Verification items for the finished model (mm, model axes). Coordinates: 2 decimals unless noted, no trailing zeros. Order: outer loops, then holes, each group sorted by start corner. A loop starts at its lowest first (then second) coordinate and runs counter-clockwise, first axis right, second up.
Q1. Cross-section at D-D, the plane x = -8.5. Record the boundary of the cut face in (y, z), and give its area (3 significant figures).
Q2. Cross-section at C-C, the plane y = 0.75. Record the boundary of the cut face in (x, z).
Q3. Thickness scan on line 1 (Y direction, x = 6, z = 6.5); line 2 (X direction, y = 1, z = 1.25); line 3 (X direction, y = 4.25, z = 1.5). Record the ranges inside material, lowest first.
Q4. Cross-section at B-B, the plane z = 8.5. Record the boundary of the cut face in (x, y), and give its area (3 significant figures).
Q5. Cross-section at A-A, the plane z = 5.75. Record the boundary of the cut face in (x, y).
Q6. Draft check along X on faces 1 (the conical face through (-4.59, -10.975, 9.604)), 2 (the flat face through (0, 0, 8)), 3 (the flat face through (5, -5, 0)), 4 (the conical face through (4.59, 10.975, 0.396)). Enter one of: pulls with the +X half, pulls with the -X half, needs draft (parallel to the pull), parting line crosses it, or undercut.
Q7. Depth check by flat-ended pin: P1, Ø4, axis at x = 0, y = -3, coming from the -Z side; P2, Ø1, axis at y = -7.5, z = 7, coming from the -X side; P3, Ø1.5, axis at y = 9, z = 3, coming from the -X side. Enter the tip coordinate at first touch or a pass-through.
from build123d import *

# Parameters (mm, degrees)
F1_DEPTH = 10
F2_DEPTH = 8
F3_SIZE  = 1


with BuildPart() as f1:
    # F0 (on Top) → F1 (new body)
    with BuildSketch(Plane.XY):
        with BuildLine():
            ThreePointArc((12.1776870536, -2.8202726863), (11.0142451748, 0), (12.1776870536, 2.8202726863))
            ThreePointArc((12.1776870536, 2.8202726863), (11.5484941564, 4.7835429046), (10.605159036, 6.6166911535))
            ThreePointArc((10.605159036, 6.6166911535), (7.7882474528, 7.7882474528), (6.6166911535, 10.605159036))
            ThreePointArc((6.6166911535, 10.605159036), (4.7835429046, 11.5484941564), (2.8202726863, 12.1776870536))
            ThreePointArc((2.8202726863, 12.1776870536), (0, 11.0142451748), (-2.8202726863, 12.1776870536))
            ThreePointArc((-2.8202726863, 12.1776870536), (-4.7835429046, 11.5484941564), (-6.6166911535, 10.605159036))
            ThreePointArc((-6.6166911535, 10.605159036), (-7.7882474528, 7.7882474528), (-10.605159036, 6.6166911535))
            ThreePointArc((-10.605159036, 6.6166911535), (-11.5484941564, 4.7835429046), (-12.1776870536, 2.8202726863))
            ThreePointArc((-12.1776870536, 2.8202726863), (-11.3165274676, 1.5254126516), (-11.0142451748, 0))
            ThreePointArc((-11.0142451748, 0), (-11.3165274676, -1.5254126516), (-12.1776870536, -2.8202726863))
            ThreePointArc((-12.1776870536, -2.8202726863), (-11.5484941564, -4.7835429046), (-10.605159036, -6.6166911535))
            ThreePointArc((-10.605159036, -6.6166911535), (-7.7882474528, -7.7882474528), (-6.6166911535, -10.605159036))
            ThreePointArc((-6.6166911535, -10.605159036), (-4.7835429046, -11.5484941564), (-2.8202726863, -12.1776870536))
            ThreePointArc((-2.8202726863, -12.1776870536), (0, -11.0142451748), (2.8202726863, -12.1776870536))
            ThreePointArc((2.8202726863, -12.1776870536), (4.7835429046, -11.5484941564), (6.6166911535, -10.605159036))
            ThreePointArc((6.6166911535, -10.605159036), (7.7882474528, -7.7882474528), (10.605159036, -6.6166911535))
            ThreePointArc((10.605159036, -6.6166911535), (11.5484941564, -4.7835429046), (12.1776870536, -2.8202726863))
        make_face()
        Polygon((6.2885942892, 3.6569908211), (6.3113440971, -3.617586998), (0.0227498078, -7.2745778191), (-6.2885942892, -3.6569908211), (-6.3113440971, 3.617586998), (-0.0227498078, 7.2745778191), align=None, mode=Mode.SUBTRACT)
        Polygon((0.0227498078, -7.2745778191), (6.3113440971, -3.617586998), (6.2885942892, 3.6569908211), (-0.0227498078, 7.2745778191), (-6.3113440971, 3.617586998), (-6.2885942892, -3.6569908211), align=None)
    extrude(amount=F1_DEPTH)

    # F0 (on Top) → F2 (cut)
    with BuildSketch(Plane.XY):
        Polygon((0.0227498078, -7.2745778191), (6.3113440971, -3.617586998), (6.2885942892, 3.6569908211), (-0.0227498078, 7.2745778191), (-6.3113440971, 3.617586998), (-6.2885942892, -3.6569908211), align=None)
    extrude(amount=F2_DEPTH, mode=Mode.SUBTRACT)

    # F3
    f3_edges = [f1.edges().sort_by_distance(p)[0] for p in [
        (11.548494, -4.783543, 10),
        (11.548494, 4.783543, 10),
        (4.783543, 11.548494, 10),
        (-4.783543, 11.548494, 10),
        (-11.548494, 4.783543, 10),
        (-11.548494, -4.783543, 10),
        (-4.783543, -11.548494, 10),
        (4.783543, -11.548494, 10),
        (4.783543, -11.548494, 0),
        (11.548494, -4.783543, 0),
        (11.548494, 4.783543, 0),
        (4.783543, 11.548494, 0),
        (-4.783543, 11.548494, 0),
        (-11.548494, 4.783543, 0),
        (-11.548494, -4.783543, 0),
        (-4.783543, -11.548494, 0),
    ]]
    chamfer(f3_edges, length=F3_SIZE)


solid = f1.part
Check values:
1. outline: (-7.22, 0) - (7.22, 0) - (7.22, 10) - (-7.22, 10) - close
1. area: 144 mm2
2. outline: (-11.09, 0) - (-6.3, 0) - (-6.3, 8) - (6.3, 8) - (6.3, 0) - (11.09, 0) - (11.09, 10) - (-11.09, 10) - close
3. line 1: y = -10.97 to -3.8, 3.82 to 10.97
3. line 2: x = -11.14 to -6.3, 6.3 to 11.14
3. line 3: x = -11.76 to -5.22, 5.25 to 11.76
4. outline: (-12.18, -2.82) arc R12.5 ccw to (-10.61, -6.62) arc R4 cw to (-6.62, -10.61) arc R12.5 ccw to (-2.82, -12.18) arc R4 cw to (2.82, -12.18) arc R12.5 ccw to (6.62, -10.61) arc R4 cw to (10.61, -6.62) arc R12.5 ccw to (12.18, -2.82) arc R4 cw to (12.18, 2.82) arc R12.5 ccw to (10.61, 6.62) arc R4 cw to (6.62, 10.61) arc R12.5 ccw to (2.82, 12.18) arc R4 cw to (-2.82, 12.18) arc R12.5 ccw to (-6.62, 10.61) arc R4 cw to (-10.61, 6.62) arc R12.5 ccw to (-12.18, 2.82) arc R4 cw to start
4. area: 445 mm2
5. outline: (-12.18, -2.82) arc R12.5 ccw to (-10.61, -6.62) arc R4 cw to (-6.62, -10.61) arc R12.5 ccw to (-2.82, -12.18) arc R4 cw to (2.82, -12.18) arc R12.5 ccw to (6.62, -10.61) arc R4 cw to (10.61, -6.62) arc R12.5 ccw to (12.18, -2.82) arc R4 cw to (12.18, 2.82) arc R12.5 ccw to (10.61, 6.62) arc R4 cw to (6.62, 10.61) arc R12.5 ccw to (2.82, 12.18) arc R4 cw to (-2.82, 12.18) arc R12.5 ccw to (-6.62, 10.61) arc R4 cw to (-10.61, 6.62) arc R12.5 ccw to (-12.18, 2.82) arc R4 cw to start; hole (-6.31, 3.62) - (-6.29, -3.66) - (0.02, -7.27) - (6.31, -3.62) - (6.29, 3.66) - (-0.02, 7.27) - close
6. face 1: pulls with the -X half
6. face 2: undercut
6. face 3: needs draft
6. face 4: pulls with the +X half
7. P1: stops at z = 8
7. P2: stops at x = -8.91
7. P3: stops at x = -7.39
